```python
from build123d import *

# Parameters (mm, degrees)
SKETCH1_R           = 6
BOSS_EXTRUDE1_DEPTH = 8
SKETCH2_OUTSIDE_W   = 84.942
SKETCH2_OUTSIDE_H   = 80.92
SKETCH2_OUTSIDE_R   = 13
CUT_EXTRUDE1_DEPTH  = 22.408720964
CUT_EXTRUDE1_DRAFT  = -45
SKETCH5_OUTSIDE_W   = 84.942
SKETCH5_OUTSIDE_H   = 80.92
SKETCH5_OUTSIDE_R   = 13
CUT_EXTRUDE2_DEPTH  = 22.408720964
CUT_EXTRUDE2_DRAFT  = -45


with BuildPart() as part:
    # Sketch1 → Boss-Extrude1 (new body)
    with BuildSketch(Plane(origin=(0, 0, 0), x_dir=(1, 0, 0), z_dir=(0, 1, 0))):
        Polygon((-15.011106999, 0), (-7.505553499, -13), (7.505553499, -13), (15.011106999, 0), (7.505553499, 13), (-7.505553499, 13), align=None)
        with Locations(Location((0, 0, 0), (0, 0, 270))):
            Circle(SKETCH1_R, mode=Mode.SUBTRACT)
    extrude(amount=BOSS_EXTRUDE1_DEPTH)


with BuildPart() as cut_extrude1_tool:
    # Sketch2 outside → Cut-Extrude1 (with draft: the straight prism first)
    with BuildSketch(Plane(origin=(0, 8, 0), x_dir=(1, 0, 0), z_dir=(0, 1, 0))):
        Rectangle(SKETCH2_OUTSIDE_W, SKETCH2_OUTSIDE_H)
        Circle(SKETCH2_OUTSIDE_R, mode=Mode.SUBTRACT)
    extrude(amount=-CUT_EXTRUDE1_DEPTH)
    # Cut-Extrude1: the draft: its side faces are tilted about the plane it starts from
    cut_extrude1_sides = [cut_extrude1_tool.faces().sort_by_distance(p)[0] for p in [
        (0, -3.204360482, 40.46),
        (42.471, -3.204360482, 0),
        (0, -3.204360482, -40.46),
        (-42.471, -3.204360482, 0),
        (-13, -3.204360482, 0),
    ]]
    draft(cut_extrude1_sides, Plane(origin=(0, 8, 0), x_dir=(1, 0, 0), z_dir=(0, 1, 0)), CUT_EXTRUDE1_DRAFT)


with BuildPart() as part_1:
    add(part.part)

    # Cut-Extrude1: cut by cut_extrude1_tool
    add(cut_extrude1_tool.part, mode=Mode.SUBTRACT)


with BuildPart() as cut_extrude2_tool:
    # Sketch5 outside → Cut-Extrude2 (with draft: the straight prism first)
    with BuildSketch(Plane(origin=(0, 0, 0), x_dir=(-1, 0, 0), z_dir=(0, -1, 0))):
        Rectangle(SKETCH5_OUTSIDE_W, SKETCH5_OUTSIDE_H)
        Circle(SKETCH5_OUTSIDE_R, mode=Mode.SUBTRACT)
    extrude(amount=-CUT_EXTRUDE2_DEPTH)
    # Cut-Extrude2: the draft: its side faces are tilted about the plane it starts from
    cut_extrude2_sides = [cut_extrude2_tool.faces().sort_by_distance(p)[0] for p in [
        (0, 11.204360482, 40.46),
        (-42.471, 11.204360482, 0),
        (0, 11.204360482, -40.46),
        (42.471, 11.204360482, 0),
        (13, 11.204360482, 0),
    ]]
    draft(cut_extrude2_sides, Plane(origin=(0, 0, 0), x_dir=(-1, 0, 0), z_dir=(0, -1, 0)), CUT_EXTRUDE2_DRAFT)


with BuildPart() as part_2:
    add(part_1.part)

    # Cut-Extrude2: cut by cut_extrude2_tool
    add(cut_extrude2_tool.part, mode=Mode.SUBTRACT)


solid = part_2.part
```
Geometry: final body of the model. Coordinates: model frame, mm. Coordinates: 2 decimals unless noted, no trailing zeros. Order: outer loops, then holes, each group sorted by start corner. A loop starts at its lowest first (then second) coordinate and runs counter-clockwise, first axis right, second up. Notation, with made-up numbers: (-38.75, 40) -> (11.25, 40) arc R26 cw to (11.25, 66) -> close; hole circle Ø11 at (79.25, -9). An arc over 180 degrees is marked (long way). Write each question's results on one line, items separated by ' | '. Start each with the question number.
1) First-contact query: pin 1 (1 mm diameter, centred on y = 6.5, z = -5.5, fed in from +X); pin 2 (1.5 mm diameter, centred on y = 1, z = -5.5, fed in from +X). Flat tips, straight axial feed; report the tip coordinate or a pass-through.
2) Material intervals for line 1 along X through (y, z) = (5.5, 2.75); line 2 along Z through (x, y) = (2, 2.25); line 3 along X through (y, z) = (6.5, 3.75), sorted ascending.
3) Cut plane A-A, the plane y = 5.25. Output: boundary loops of the cut face in (x, z), and give its area (3 significant figures).
4) Mould query, pull axis X, two halves, no side actions, for faces 1 (the flat face through (-11.2, 3.9, -6.6)), 2 (the cylindrical face through (1.802, 3.944, 5.723)), 3 (the flat face through (0, 4, 13)). Classes: released by +X, released by -X, zero draft, split by the parting line, or undercut.
Checks:
1) pin 1: x = 12.12 | pin 2: x = 12.27
2) line 1: -13.42 to -5.33, 5.33 to 13.42 | line 2: -13 to -5.66, 5.66 to 13 | line 3: -12.85 to -4.68, 4.68 to 12.85
3) outline: (-15.01, 0) -> (-7.51, -13) -> (7.51, -13) -> (15.01, 0) -> (7.51, 13) -> (-7.51, 13) -> close; hole circle Ø12 at (0, 0) | area: 472 mm^2
4) face 1: released by -X | face 2: undercut | face 3: zero draft
